Part model, mm, in its own coordinate system. Face numbers are marked on the shaded views. A direction names the side the tool comes from. Give positions to 0.01 mm unless a question says otherwise; leave off trailing zeros. Order: outer loops, then holes, each group sorted by start corner. A loop starts at its lowest first (then second) coordinate and runs counter-clockwise, first axis right, second up. Notation, with made-up numbers: M 69.25,-11 L 98.25,-11 A16 cw 98.25,-6 Z; hole C 0,66.25 d9. An arc over 180 degrees is marked long. Answer as a JSON object with one key per item and string values.
from build123d import *

# Parameters (mm, degrees)
PAD_DEPTH = 490
FILLET_R  = 18


with BuildPart() as part:
    # Sketch → Pad (new body)
    with BuildSketch(Plane.XZ):
        Polygon((0, 0), (150, 0), (150, 80), (0, 80), (-13, 80), (-13, -20), (0, -20), align=None)
    extrude(amount=-PAD_DEPTH)

    # Fillet
    fillet_edges = [part.edges().sort_by_distance(p)[0] for p in [
        (-13, 245, 80),
    ]]
    fillet(fillet_edges, radius=FILLET_R)


solid = part.part
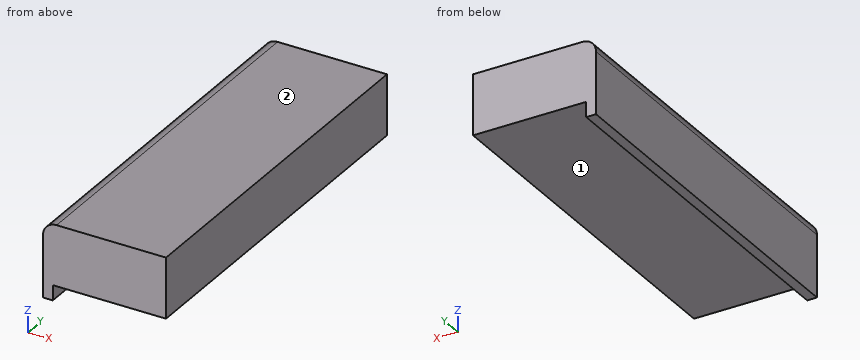
1. Probe line 1 along X through (y, z) = (93.5, -5); line 2 along Z through (x, y) = (64, 144); line 3 along X through (y, z) = (396, 74.5). List the from-to ranges inside material, lowest first.
Worked answers:
{"line 1": "x = -13 to 0", "line 2": "z = 0 to 80", "line 3": "x = -7.95 to 150"}
2. Which spindle directions (+Z, -Z, +X, -X, +Y, -Y) get a long thin tool onto all of the face, cutting with end or side? Do the marked faces 1 and 2. Say none if no direction does.
Worked answers:
{"face 1": "-Z, +X, +Y, -Y", "face 2": "+Z, +X, -X, +Y, -Y"}
3. Cut at B-B on x = 125.5. Give the cut face in (y, z).
Worked answers:
{"outline": "M 0,0 L 490,0 L 490,80 L 0,80 Z"}
4. Cut at A-A on y = 432. Give the cut face in (x, z).
Worked answers:
{"outline": "M -13,-20 L 0,-20 L 0,0 L 150,0 L 150,80 L 5,80 A18 ccw -13,62 Z"}
5. Pin check, flat tips, straight feed: P1, Ø2, axis at x = 67, y = 336.5, coming from the -Z side; P2, Ø16, axis at y = 291.5, z = -9.5, coming from the +X side. Stop position of each tip, or through.
Worked answers:
{"P1": "stops at z = 0", "P2": "stops at x = 0"}
6. Cut at C-C on z = -13.5. Give the cut face in (x, y).
Worked answers:
{"outline": "M -13,0 L 0,0 L 0,490 L -13,490 Z"}
